Autodesk Inventor part; units mm, degrees
ref_plane "YZ Plane" through (0, 0, 0) normal (1, 0, 0) x (0, 1, 0)
ref_plane "XZ Plane" through (0, 0, 0) normal (0, 1, 0) x (-1, 0, 0)
ref_plane "XY Plane" through (0, 0, 0) normal (0, 0, 1) x (1, 0, 0)
sketch "Szkic1" plane through (0, 0, 0) normal (0, 0, 1) x (1, 0, 0)
  line L0 (-24.8894, -0.3525) -> (25.4856, -0.3525)
  line L1 (-22.6958, -0.3525) -> (-22.6958, 4.6475)
  line L2 (-22.6958, 4.6475) -> (-17.6958, 4.6475)
  line L3 (-17.6958, 4.6475) -> (-17.6958, 5.5475)
  line L4 (-17.6958, 5.5475) -> (-15.5558, 5.5475)
  line L5 (-15.5558, 5.5475) -> (-15.5558, 2.0975)
  line L6 (-15.5558, 2.0975) -> (-11.5558, 2.0975)
  line L7 (-11.5558, 2.0975) -> (-11.5558, 5.5475)
  line L8 (-11.5558, 5.5475) -> (-9.3558, 5.5475)
  line L9 (-9.3558, 5.5475) -> (-9.3558, 4.4625)
  line L10 (-9.3558, 4.4625) -> (-3.2506, 4.4625) construction
  line L11 (-3.2506, 4.4625) -> (0.6286, 3.2981) construction
  line L12 (0.6286, 3.2981) -> (3.3042, 1.1615) construction
  line L13 (3.3042, 1.1615) -> (3.3042, -0.3525) construction
  spline S0 degree 4 poles (-9.3558, 4.4625) (-3.2506, 4.4625) (0.6286, 3.2981) (3.3042, 1.1615) (3.3042, -0.3525) knots 1 1 1 1 1 2 2 2 2 2
  point P0 (0, 0)
  point P1 (-16.6258, 5.5475)
  point P2 (-10.4558, 5.5475)
  dimension "d0" = 10
  dimension "d1" = 5
  dimension "d2" = 11.8
  dimension "d3" = 7.14
  dimension "d4" = 4.9
  dimension "d5" = 4
  dimension "d6" = 2.2
  dimension "d7" = 9.63
  dimension "d8" = 26
revolve "Obrót1" add sketch "Szkic1" angle 360 about axis through (-24.8894, -0.3525, 0) along (1, 0, 0)
fillet "Zaokrąglenie1" radius 0.5 2 edges at (-9.3558, -5.1675, 0) (-17.6958, -5.3525, 0)
sketch "Szkic2" plane through (-22.6958, -0.3525, 0) normal (-1, 0, 0) x (0, 0, 1)
  point P0 (0, 0.3525)
  point P1 (0, 0.3525)
hole "Otwór1" at (-22.6958, 0, 0) direction (1, 0, 0) diameter 3.11 depth 9 tip angle 118
properties part number "mocowanie_smigla"
Can you work these out from the model? Positions are in its coordinate system, mm. A direction names the side the tool comes from. Round coordinates to 2 decimals unless told otherwise and drop trailing zeros.
Item 1: If we mould it in two halves opening along Z, with no side actions, what happens to faces 4 (the cylindrical face through (-16.611, 5.275, 1.772)), 5 (the flat face through (-9.356, -3, -5)), 6 (the conical face through (-12.924, 0.081, 0.258))? For each: +Z half, -Z half, draft (parallel to the pull), parting line (faces both ways), or undercut.
Item 2: Please list where these lines run through material, in increasing order: L1, parallel to Z at x = -20, y = 0 (3 decimals); L2, parallel to Z at x = -16.25, y = 0 (3 decimals); L3, parallel to X at y = 2.75, z = 2.
Item 3: Which directions (+Z, -Z, +X, -X, +Y, -Y) give clear straight access to the entire face, cutting with the end or side of a thin tool? Please do faces 1 (the flat face through (-15.556, 0, -3)), 2 (the cylindrical face through (-10.44, 5.275, 1.772)), 3 (the flat face through (-17.696, -3, 5)).
Item 4: Will these pins go through, and if not, where does the flat tip stop? pin 1 Ø5 at (y, z) = (2.5, 3.5) entering from +X; pin 2 Ø5 at (y, z) = (0, 2.5) entering from +X; pin 3 Ø3.5 at (y, z) = (1.5, -2) entering from +X; pin 4 Ø2 at (x, y) = (-8, -4) entering from -Z.
Reported:
1. face 4: parting line
1. face 5: draft
1. face 6: undercut
2. L1: z = -4.988 to -1.555, 1.555 to 4.988
2. L2: z = -5.889 to -1.555, 1.555 to 5.889
2. L3: x = -22.7 to -15.56, -11.56 to -1.25
3. face 1: none
3. face 2: +X, -X
3. face 3: -X
4. pin 1: stops at x = 1.97
4. pin 2: stops at x = 3.3
4. pin 3: stops at x = 2.96
4. pin 4: stops at z = -4
